Autodesk Inventor part; units mm, degrees
ref_plane "YZ Plane" through (0, 0, 0) normal (1, 0, 0) x (0, 1, 0)
ref_plane "XZ Plane" through (0, 0, 0) normal (0, 1, 0) x (-1, 0, 0)
ref_plane "XY Plane" through (0, 0, 0) normal (0, 0, 1) x (1, 0, 0)
sketch "Sketch1" plane through (0, 0, 0) normal (0, 0, 1) x (1, 0, 0)
  line L0 (0, 0) -> (150, 0)
  line L1 (150, 0) -> (150, -150)
  line L2 (150, -150) -> (0, -150)
  line L3 (0, -150) -> (0, 0)
  circle A0 centre (75, -75) radius 12.5
  dimension "d0" = 150
  dimension "d1" = 150
  dimension "d2" = 25
  dimension "d3" = 75
  dimension "d4" = 75
extrude "Extrusion1" add sketch "Sketch1" along normal blind 3
ref_plane "Work Plane3" through (0, -75, 0) normal (0, 1, 0) x (1, 0, 0)
ref_plane "Work Plane4" through (75, -150, 0) normal (1, 0, 0) x (0, 0, -1)
properties part number "box" material "ABS Plastic"
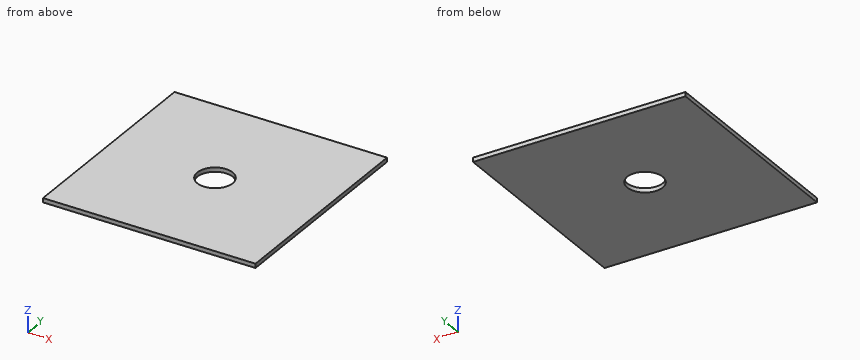
Model file for the job. Use its own axes, mm. Round coordinates to 2 decimals unless told otherwise and drop trailing zeros. Loops run counter-clockwise (first coordinate to the right, second up) from the corner with the lowest first, then second, coordinate; pieces in that order, holes last. Notation, with made-up numbers: M 32.25,-25 L 53.25,-25 A18 cw 53.25,-3 Z; hole C 28,33.5 d6. An arc over 180 degrees is marked long. Put each result on its own line as item: value. Start each with the question number.
Item 1: Cut at C-C (z = 2.25). List the corners of the cut face in (x, y), then the cut area to 3 significant figures.
Item 2: Drill centre lines: line 1 along Y through (x, z) = (75, 1.7); line 2 along Y through (x, z) = (71, 1.3); line 3 along X through (y, z) = (-80.5, 0.4). Where is each one in solid material? Low to high.
Item 3: Cut at A-A (y = -75). List the corners of the cut face in (x, z), then the cut area to 3 significant figures.
Item 4: Drop a flat-ended pin along its axis: P1, Ø22.5, axis at x = 75, y = -75, coming from the +Z side. Give the stop position or say it passes through.
Item 5: Cut at B-B (x = 75). List the corners of the cut face in (y, z).
Answer block:
1. outline: M 0,-150 L 150,-150 L 150,0 L 0,0 Z; hole C 75,-75 d25
1. area: 22,000 mm2
2. line 1: -150 to -87.5, -62.5 to 0
2. line 2: -150 to -86.84, -63.16 to 0
2. line 3: 0 to 63.78, 86.22 to 150
3. outline: M 0,0 L 62.5,0 L 62.5,3 L 0,3 Z; M 87.5,0 L 150,0 L 150,3 L 87.5,3 Z
3. area: 375 mm2
4. P1: through
5. outline: M -150,0 L -87.5,0 L -87.5,3 L -150,3 Z; M -62.5,0 L 0,0 L 0,3 L -62.5,3 Z
